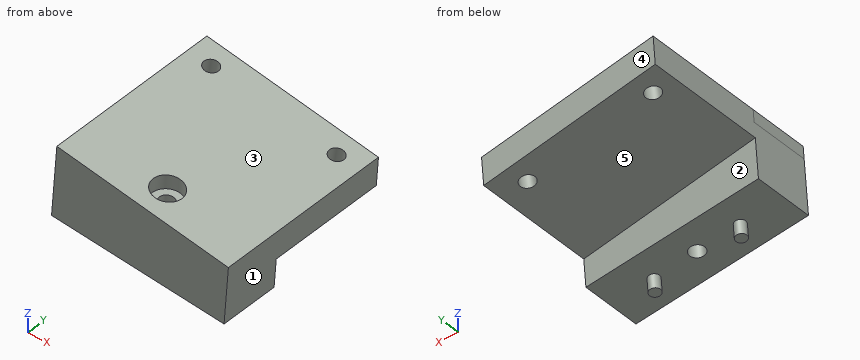
from build123d import *

# Parameters (mm, degrees)
BOSS_EXTRUDE1_OUTLINE_W   = 76.2
BOSS_EXTRUDE1_OUTLINE_H   = 25.4
BOSS_EXTRUDE1_OUTLINE_R   = 3.2639
BOSS_EXTRUDE1_DEPTH       = 25.471337323
BOSS_EXTRUDE1_START       = -25.4
BOSS_EXTRUDE1_2_DEPTH     = 25.4
BOSS_EXTRUDE1_START_2     = 333.890252769
BOSS_EXTRUDE1_3_OUTLINE_R = 3.2639
BOSS_EXTRUDE1_3_DEPTH     = 5.715
BOSS_EXTRUDE2_START       = 302.068915446
BOSS_EXTRUDE2_OUTLINE_R   = 2.3622
BOSS_EXTRUDE2_DEPTH       = 6.931084554
BOSS_EXTRUDE3_DEPTH       = 50.8
SKETCH6_R                 = 3.19999995
CUT_EXTRUDE1_DEPTH        = 120.033223303
SKETCH8_R                 = 6.35
CUT_EXTRUDE2_DEPTH        = 6.35


with BuildPart() as part:
    # Boss-Extrude1: read off the stored shape, not the designer's step
    # Boss-Extrude1 outline → Boss-Extrude1 (new body)
    with BuildSketch(Plane(origin=(23.066634723, 0, 307.55512964), x_dir=(0.9971993098884564, 0, -0.07478994824163422), z_dir=(0.07478994824163422, 0, 0.9971993098884564))):
        with Locations((38.1, -12.7)):
            Rectangle(BOSS_EXTRUDE1_OUTLINE_W, BOSS_EXTRUDE1_OUTLINE_H)
        with Locations((38.1, -12.701750828)):
            Circle(BOSS_EXTRUDE1_OUTLINE_R, mode=Mode.SUBTRACT)
    extrude(amount=BOSS_EXTRUDE1_DEPTH)

    # Boss-Extrude1 2 outline → Boss-Extrude1 2 (add)
    with BuildSketch(Plane(origin=(0, 0, 0), x_dir=(1, 0, 0), z_dir=(0, 1, 0)).offset(BOSS_EXTRUDE1_START)):
        Polygon((101.385646691, -332.95512964), (100.958222137, -327.256135584), (24.971634723, -332.95512964), align=None)
    extrude(amount=BOSS_EXTRUDE1_2_DEPTH)

    # Boss-Extrude1 3 outline → Boss-Extrude1 3 (cut)
    with BuildSketch(Plane(origin=(0, 0, 0), x_dir=(0.9971993098884564, 0, -0.07478994824163422), z_dir=(0.07478994824163422, 0, 0.9971993098884564)).offset(BOSS_EXTRUDE1_START_2)):
        with Locations((38.1, -12.701750828)):
            Circle(BOSS_EXTRUDE1_3_OUTLINE_R)
    extrude(amount=BOSS_EXTRUDE1_3_DEPTH, mode=Mode.SUBTRACT)

    # Boss-Extrude2: read off the stored shape, not the designer's step
    # Boss-Extrude2 outline → Boss-Extrude2 (add)
    with BuildSketch(Plane(origin=(0, 0, 0), x_dir=(0.9971993098884564, 0, -0.07478994824163422), z_dir=(0.07478994824163422, 0, 0.9971993098884564)).offset(BOSS_EXTRUDE2_START)):
        with Locations((57.15, -12.701750828)):
            Circle(BOSS_EXTRUDE2_OUTLINE_R)
        with Locations((19.05, -12.701750828)):
            Circle(BOSS_EXTRUDE2_OUTLINE_R)
    extrude(amount=BOSS_EXTRUDE2_DEPTH)

    # Sketch7 → Boss-Extrude3 (add)
    with BuildSketch(Plane(origin=(0, 0, 0), x_dir=(1, 0, 0), z_dir=(0, 1, 0))):
        Polygon((24.971634723, -332.95512964), (24.019134723, -320.25512964), (100.433146691, -320.25512964), (101.385646691, -332.95512964), align=None)
    extrude(amount=BOSS_EXTRUDE3_DEPTH)

    # Sketch6 → Cut-Extrude1 (cut, through all)
    with BuildSketch(Plane.XY.offset(332.95512964)):
        with Locations((35.238640707, 41.275)):
            Circle(SKETCH6_R)
        with Locations((91.118640707, 41.275)):
            Circle(SKETCH6_R)
    extrude(amount=-CUT_EXTRUDE1_DEPTH, mode=Mode.SUBTRACT)

    # Sketch8 → Cut-Extrude2 (cut)
    with BuildSketch(Plane(origin=(25.220865956, 0, 336.278212746), x_dir=(-0.9971993098884564, 0, 0.07478994824163424), z_dir=(-0.07478994824163424, 0, -0.9971993098884564))):
        with Locations(Location((-38.1, -12.701750828, 0), (0, 0, 175.710846671))):
            Circle(SKETCH8_R)
    extrude(amount=CUT_EXTRUDE2_DEPTH, mode=Mode.SUBTRACT)


with BuildPart() as body_2:
    # Mirror1: mirrored copy
    add(part.part.mirror(Plane(origin=(107.187637483, 0, 410.315006871), x_dir=(0.07478994824163424, 0, 0.9971993098884564), z_dir=(-0.9971993098884564, 1.0351948349208248e-14, 0.07478994824163424))))


solid = body_2.part
Model file for the job. Use its own axes, mm. Face numbers are marked on the shaded views. A direction names the side the tool comes from. Round coordinates to 2 decimals unless told otherwise and drop trailing zeros. Loops run counter-clockwise (first coordinate to the right, second up) from the corner with the lowest first, then second, coordinate; pieces in that order, holes last. Notation, with made-up numbers: M 56,-7 L 66,-7 A26 cw 66,9 Z; hole C -29,64 d5. An arc over 180 degrees is marked long. One line per question, with ' | ' between items.
1) Band-saw the part on D-D (z = 313.5). Give the number of separate pieces and of enclosed holes in the cut face, then the cut area to 3 significant figures.
Solved:
separate pieces: 1 | enclosed holes: 2 | area: 3,460 mm²
2) Flat gauge pins, fed straight in: pin 1 (5 mm diameter, centred on x = 110, y = 25, fed in from -Z); pin 2 (3 mm diameter, centred on x = 146, z = 328.5, fed in from -Y); pin 3 (1.5 mm diameter, centred on x = 134.5, y = -11.5, fed in from -Z); pin 4 (2 mm diameter, centred on x = 124.5, y = 13, fed in from +Z). Where does each tip first touch, or does it go through?
Solved:
pin 1: stops at z = 318.43 | pin 2: passes through | pin 3: stops at z = 299.2 | pin 4: stops at z = 329.62
3) Drill centre lines: line 1 along Y through (x, z) = (113, 310); line 2 along Y through (x, z) = (137.5, 314); line 3 along Z through (x, y) = (125, 30). Where is each one in solid material? Low to high.
Solved:
line 1: y = -25.4 to 0 | line 2: y = -25.4 to -15.9, -9.51 to 0 | line 3: z = 316.55 to 329.39
4) Mould opens along Z. For the marked faces 3, 4 and 5 say: +Z half, -Z half, draft (parallel to the pull), parting line (faces both ways), or undercut.
Solved:
face 3: +Z half | face 4: draft | face 5: -Z half
5) Band-saw the part on B-B (x = 149). Give the cut face in (y, z).
Solved:
outline: M -25.4,298.11 L 0,298.11 L 0,312.93 L 50.8,312.93 L 50.8,325.77 L -25.4,325.77 Z
6) Band-saw the part on A-A (y = 40). Give the cut face in (x, z), then the cut area to 3 significant figures.
Solved:
outline: M 100.43,320.26 L 106.74,319.3 L 108.64,331.86 L 101.39,332.96 Z; M 112.55,318.43 L 162,310.97 L 163.89,323.53 L 114.44,330.99 Z; M 167.8,310.09 L 175.99,308.86 L 176.94,321.56 L 169.69,322.65 Z | area: 821 mm²
7) 3-axis set-ups, long thin cutter, end or side, ignore diameter. For the marked faces 1 and 2: which of +Z, -Z, +X, -X, +Y, -Y reach the whole face in a straight line?
Solved:
face 1: -Z, +X, +Y, -Y | face 2: -Z, -X, +Y
8) Band-saw the part on C-C (y = -7.5). Give the cut face in (x, z), then the cut area to 3 significant figures.
Solved:
outline: M 99.05,301.86 L 175.04,296.16 L 176.94,321.56 L 142.78,326.71 L 142.36,321.13 L 135.09,321.67 L 135.55,327.8 L 101.39,332.96 Z | area: 2,120 mm²
